The listing builds one solid part. Answer for the finished solid, in the listing's coordinates (mm). A direction names the side the tool comes from. Coordinates: 2 decimals unless noted, no trailing zeros. Order: outer loops, then holes, each group sorted by start corner. A loop starts at its lowest first (then second) coordinate and runs counter-clockwise, first axis right, second up. Notation, with made-up numbers: (-19.75, 36) -> (7.25, 36) arc R28 cw to (7.25, 61) -> close; hole circle Ø10 at (-22, 22). An arc over 180 degrees is marked (long way). One line per question, with ' | ' between items.
from build123d import *

# Parameters (mm, degrees)
PAD_DEPTH = 50


with BuildPart() as part:
    # Sketch → Pad (new body)
    with BuildSketch(Plane.XY):
        with BuildLine():
            Line((0, 17.2), (0, 0))
            Line((0, 0), (17.2, 0))
            ThreePointArc((17.2, 0), (17.765685, 0.234315), (18, 0.8))
            Line((18, 0.8), (18, 2))
            Line((18, 2), (2.6, 2))
            ThreePointArc((2, 2.6), (1.575736, 1.575736), (2.6, 2))
            Line((2, 2.6), (2, 18))
            Line((2, 18), (0.8, 18))
            ThreePointArc((0.8, 18), (0.234315, 17.765685), (0, 17.2))
        make_face()
    extrude(amount=PAD_DEPTH)


solid = part.part
Item 1: Section B-B, the plane x = 9.25 is taken. Give the vertices of the cut face in (y, z).
Computed values:
outline: (0, 0) -> (2, 0) -> (2, 50) -> (0, 50) -> close
Item 2: Find the intervals of material crossed by L1, parallel to X at y = 8.75, z = 8; L2, parallel to X at y = 1.5, z = 36, in increasing order.
Computed values:
L1: x = 0 to 2 | L2: x = 0 to 1.67, 2.33 to 18
Item 3: For faces 5 (the face through (0, 9, 25)), 6 (the face through (10, 2, 25)), determine the directions among +Z, -Z, +X, -X, +Y, -Y from which every point of the face is accessible in a straight line to the end or side of a thin tool.
Computed values:
face 5: +Z, -Z, -X, +Y, -Y | face 6: +Z, -Z, +X, +Y
Item 4: Each of these flat-tipped pins is pushed along its axis until it touches: pin 1 Ø1.5 at (y, z) = (9.5, 34.5) entering from +X; pin 2 Ø8 at (x, y) = (10.5, 5.5) entering from -Z; pin 3 Ø1 at (x, y) = (2, 2) entering from +Z. Where does it stop, or does it pass through?
Computed values:
pin 1: stops at x = 2 | pin 2: stops at z = 0 | pin 3: passes through
Item 5: Section A-A, the plane z = 38.5 is taken. Give the vertices of the cut face in (x, y).
Computed values:
outline: (0, 0) -> (17.2, 0) arc R0.8 ccw to (18, 0.8) -> (18, 2) -> (2.6, 2) arc R0.6 cw (long way) to (2, 2.6) -> (2, 18) -> (0.8, 18) arc R0.8 ccw to (0, 17.2) -> close
Item 6: Determine the mould class of faces 1 (the face through (1.56, 1.59, 24.65)), 2 (the face through (1.6, 5.7, 50)), 3 (the face through (8, 0, 25)), 4 (the face through (1, 18, 25)) for opening direction Y: pulls with the +Y half, pulls with the -Y half, needs draft (parallel to the pull), parting line crosses it, or undercut.
Computed values:
face 1: undercut | face 2: needs draft | face 3: pulls with the -Y half | face 4: pulls with the +Y half
